Can you work these out from the model? Positions are in its coordinate system, mm. A direction names the side the tool comes from. Coordinates: 2 decimals unless noted, no trailing zeros. Write each loop counter-clockwise with the first axis right and the second up, starting at its lowest first coordinate (ties: lowest second). Pieces come first, ordered by that corner, then holes. Notation, with made-up numbers: (29.25, -17) - (69.25, -17) arc R21 ccw to (69.25, 15) - close; hole circle Ø7 at (55, 16). An arc over 180 degrees is marked (long way). Write each question's results on one line, items separated by ' | '. Start each with the question number.
```python
from build123d import *

# Parameters (mm, degrees)
BOSS_EXTRUDE5_DEPTH = 4.7625
BOSS_EXTRUDE6_DEPTH = 4.7625


with BuildPart() as part:
    # Sketch1 → Boss-Extrude5 (new body)
    with BuildSketch(Plane.XY):
        with BuildLine():
            Line((0, 28.302), (0, 30.5))
            Line((0, 30.5), (-5.08, 30.5))
            Line((-5.08, 30.5), (-5.08, 5.08))
            Line((-5.08, 5.08), (0, 5.08))
            Line((0, 5.08), (0, 21.698))
            ThreePointArc((0, 21.698), (-3.302, 25), (0, 28.302))
        make_face()
        with BuildLine():
            Line((5.08, 30.5), (0, 30.5))
            Line((0, 30.5), (0, 28.302))
            ThreePointArc((0, 28.302), (2.334866591, 27.334866591), (3.302, 25))
            ThreePointArc((3.302, 25), (2.334866591, 22.665133409), (0, 21.698))
            Line((0, 21.698), (0, 5.08))
            Line((0, 5.08), (5.08, 5.08))
            Line((5.08, 5.08), (5.08, 30.5))
        make_face()
        with BuildLine():
            Line((30.5, 5.08), (5.08, 5.08))
            Line((5.08, 5.08), (5.08, 2.171785995))
            ThreePointArc((5.08, 2.171785995), (6.282811882, 1.369173548), (6.7479, 0))
            Line((6.7479, 0), (22.2521, 0))
            ThreePointArc((22.2521, 0), (24.5, 2.2479), (26.7479, 0))
            Line((26.7479, 0), (30.5, 0))
            Line((30.5, 0), (30.5, 5.08))
        make_face()
        with BuildLine():
            Line((22.2521, 0), (6.7479, 0))
            ThreePointArc((6.7479, 0), (6.282811882, -1.369173548), (5.08, -2.171785995))
            Line((5.08, -2.171785995), (5.08, -5.08))
            Line((5.08, -5.08), (30.5, -5.08))
            Line((30.5, -5.08), (30.5, 0))
            Line((30.5, 0), (26.7479, 0))
            ThreePointArc((26.7479, 0), (24.5, -2.2479), (22.2521, 0))
        make_face()
        with BuildLine():
            Line((2.2521, 0), (0, 0))
            Line((0, 0), (0, -5.08))
            Line((0, -5.08), (5.08, -5.08))
            Line((5.08, -5.08), (5.08, -2.171785995))
            ThreePointArc((5.08, -2.171785995), (3.130826452, -1.782811882), (2.2521, 0))
        make_face()
        with BuildLine():
            Line((0, -5.08), (0, 0))
            Line((0, 0), (-2.2521, 0))
            ThreePointArc((-2.2521, 0), (-3.130826452, -1.782811882), (-5.08, -2.171785995))
            Line((-5.08, -2.171785995), (-5.08, -5.08))
            Line((-5.08, -5.08), (0, -5.08))
        make_face()
        with BuildLine():
            Line((5.08, 2.171785995), (5.08, 5.08))
            Line((5.08, 5.08), (0, 5.08))
            Line((0, 5.08), (0, 0))
            Line((0, 0), (2.2521, 0))
            ThreePointArc((2.2521, 0), (3.130826452, 1.782811882), (5.08, 2.171785995))
        make_face()
        with BuildLine():
            Line((0, 5.08), (-5.08, 5.08))
            Line((-5.08, 5.08), (-5.08, 2.171785995))
            ThreePointArc((-5.08, 2.171785995), (-3.130826452, 1.782811882), (-2.2521, 0))
            Line((-2.2521, 0), (0, 0))
            Line((0, 0), (0, 5.08))
        make_face()
        with BuildLine():
            Line((-5.08, 2.171785995), (-5.08, 5.08))
            Line((-5.08, 5.08), (-30.5, 5.08))
            Line((-30.5, 5.08), (-30.5, 0))
            Line((-30.5, 0), (-26.7479, 0))
            ThreePointArc((-26.7479, 0), (-24.5, 2.2479), (-22.2521, 0))
            Line((-22.2521, 0), (-6.7479, 0))
            ThreePointArc((-6.7479, 0), (-6.282811882, 1.369173548), (-5.08, 2.171785995))
        make_face()
        with BuildLine():
            ThreePointArc((-5.08, -2.171785995), (-6.282811882, -1.369173548), (-6.7479, 0))
            Line((-6.7479, 0), (-22.2521, 0))
            ThreePointArc((-22.2521, 0), (-24.5, -2.2479), (-26.7479, 0))
            Line((-26.7479, 0), (-30.5, 0))
            Line((-30.5, 0), (-30.5, -5.08))
            Line((-30.5, -5.08), (-5.08, -5.08))
            Line((-5.08, -5.08), (-5.08, -2.171785995))
        make_face()
        with BuildLine():
            Line((0, -21.698), (0, -5.08))
            Line((0, -5.08), (-5.08, -5.08))
            Line((-5.08, -5.08), (-5.08, -30.5))
            Line((-5.08, -30.5), (0, -30.5))
            Line((0, -30.5), (0, -28.302))
            ThreePointArc((0, -28.302), (-3.302, -25), (0, -21.698))
        make_face()
        with BuildLine():
            Line((5.08, -5.08), (0, -5.08))
            Line((0, -5.08), (0, -21.698))
            ThreePointArc((0, -21.698), (2.334866591, -22.665133409), (3.302, -25))
            ThreePointArc((3.302, -25), (2.334866591, -27.334866591), (0, -28.302))
            Line((0, -28.302), (0, -30.5))
            Line((0, -30.5), (5.08, -30.5))
            Line((5.08, -30.5), (5.08, -5.08))
        make_face()
    extrude(amount=BOSS_EXTRUDE5_DEPTH)

    # Sketch3 → Boss-Extrude6 (add)
    with BuildSketch(Plane.XY.offset(4.7625)):
        Polygon((5.08, 5.08), (15.748, 5.08), (5.08, 15.748), align=None)
        Polygon((5.08, -5.08), (5.08, -15.748), (15.748, -5.08), align=None)
        Polygon((-5.08, -5.08), (-15.748, -5.08), (-5.08, -15.748), align=None)
        Polygon((-15.748, 5.08), (-5.08, 5.08), (-5.08, 15.748), align=None)
    extrude(amount=-BOSS_EXTRUDE6_DEPTH)


solid = part.part
```
Q1. If we section it at D-D (y = 17): Please give me the cut outline in (x, z), then the cut area to 3 significant figures.
Q2. If we section it at A-A (x = -24.5): Please give me the cut outline in (y, z), then the cut area to 3 significant figures.
Q3. If we section it at B-B (z = 3.8): Please give me the cut outline in (x, y), then the cut area to 3 significant figures.
Q4. Thinking about a two-plate mould opening in X: for faces 1 (the face through (-10.34, 10.49, 2.41)), 2 (the face through (5.08, 23, 2)), 3 (the face through (22.254, -0.099, 2.348)), which applies, pulls with the +X half, pulls with the -X half, needs draft (parallel to the pull), parting line crosses it, or undercut?
Q5. I'm going to push flat-ended pins straight in: pin 1 Ø1.4 at (y, z) = (26.5, 2.5) entering from -X; pin 2 Ø1.4 at (y, z) = (21.5, 2.5) entering from +X. Where does each tip first touch, or does it pass through?
Q6. For faces 4 (the face through (23, -5.08, 2)), 5 (the face through (-23, 5.08, 2)), 6 (the face through (-5.08, -23, 2)), which set-ups out of +Z, -Z, +X, -X, +Y, -Y let a thin tool reach every point of the face, with its end or its side?
Q7. If we section it at C-C (y = -26): Please give me the cut outline in (x, z).
Q8. I need wall thicknesses on line 1 along Y through (x, z) = (24.5, 3.1); line 2 along X through (y, z) = (-0.5, 1.15); line 3 along Y through (x, z) = (1.5, 0.3). Which ranges of each line are inside material? Lowest first, please. Write a range as from..to.
Answer list:
1) outline: (-5.08, 0) - (5.08, 0) - (5.08, 4.76) - (-5.08, 4.76) - close | area: 48.4 mm2
2) outline: (-5.08, 0) - (-2.25, 0) - (-2.25, 4.76) - (-5.08, 4.76) - close; (2.25, 0) - (5.08, 0) - (5.08, 4.76) - (2.25, 4.76) - close | area: 27.0 mm2
3) outline: (-30.5, -5.08) - (-15.75, -5.08) - (-5.08, -15.75) - (-5.08, -30.5) - (5.08, -30.5) - (5.08, -15.75) - (15.75, -5.08) - (30.5, -5.08) - (30.5, 5.08) - (15.75, 5.08) - (5.08, 15.75) - (5.08, 30.5) - (-5.08, 30.5) - (-5.08, 15.75) - (-15.75, 5.08) - (-30.5, 5.08) - close; hole circle Ø4.5 at (-24.5, 0); hole circle Ø4.5 at (-4.5, 0); hole circle Ø6.6 at (0, -25); hole circle Ø6.6 at (0, 25); hole circle Ø4.5 at (4.5, 0); hole circle Ø4.5 at (24.5, 0) | area: 1,230 mm2
4) face 1: pulls with the -X half | face 2: pulls with the +X half | face 3: undercut
5) pin 1: stops at x = -5.08 | pin 2: stops at x = 5.08
6) face 4: +Z, -Z, +X, -Y | face 5: +Z, -Z, -X, +Y | face 6: +Z, -Z, -X, -Y
7) outline: (-5.08, 0) - (-3.15, 0) - (-3.15, 4.76) - (-5.08, 4.76) - close; (3.15, 0) - (5.08, 0) - (5.08, 4.76) - (3.15, 4.76) - close
8) line 1: y = -5.08..-2.25, 2.25..5.08 | line 2: x = -30.5..-26.69, -22.31..-6.69, -2.31..2.31, 6.69..22.31, 26.69..30.5 | line 3: y = -30.5..-27.94, -22.06..22.06, 27.94..30.5
